The figure shows three views and two pictorial views of one solid part (mm, origin at its lowest corner). Answer the questions. A direction names the side the tool comes from. Coordinates: 2 decimals unless noted, no trailing zeros. Loops run counter-clockwise (first coordinate to the right, second up) from the corner with the lowest first, then second, coordinate; pieces in that order, holes last. Notation, with made-up numbers: M 72.25,32 L 80.25,32 A20 cw 80.25,60 Z; hole C 81,-8.5 d11. An arc over 180 degrees is marked long. One line per item, written item: value. Start each with the question number.
1. The part is cut by section A-A (y = 40.5). Write down the section's boundary in (x, z), then the cut area to 3 significant figures.
2. The part is cut by section B-B (z = 57.5). Write down the section's boundary in (x, y).
3. Consider probe 1 along X at (y, z) = (5.5, 34.5). Determine where the line is inside the solid, lowest interval first.
4. Flat-ended cylindrical pins translate along their axes: pin 1 (24 mm diameter, centred on y = 28.5, z = 66.5, fed in from -X); pin 2 (1.2 mm diameter, centred on x = 81, y = 34.5, fed in from +Z); pin 3 (14.5 mm diameter, centred on y = 39, z = 70, fed in from +X). Find the tip coordinate at first contact, or state that the pin passes through.
5. For the marked faces 1, 2 and 3, determine the directions among +Z, -Z, +X, -X, +Y, -Y from which every point of the face is accessible in a straight line to the end or side of a thin tool.
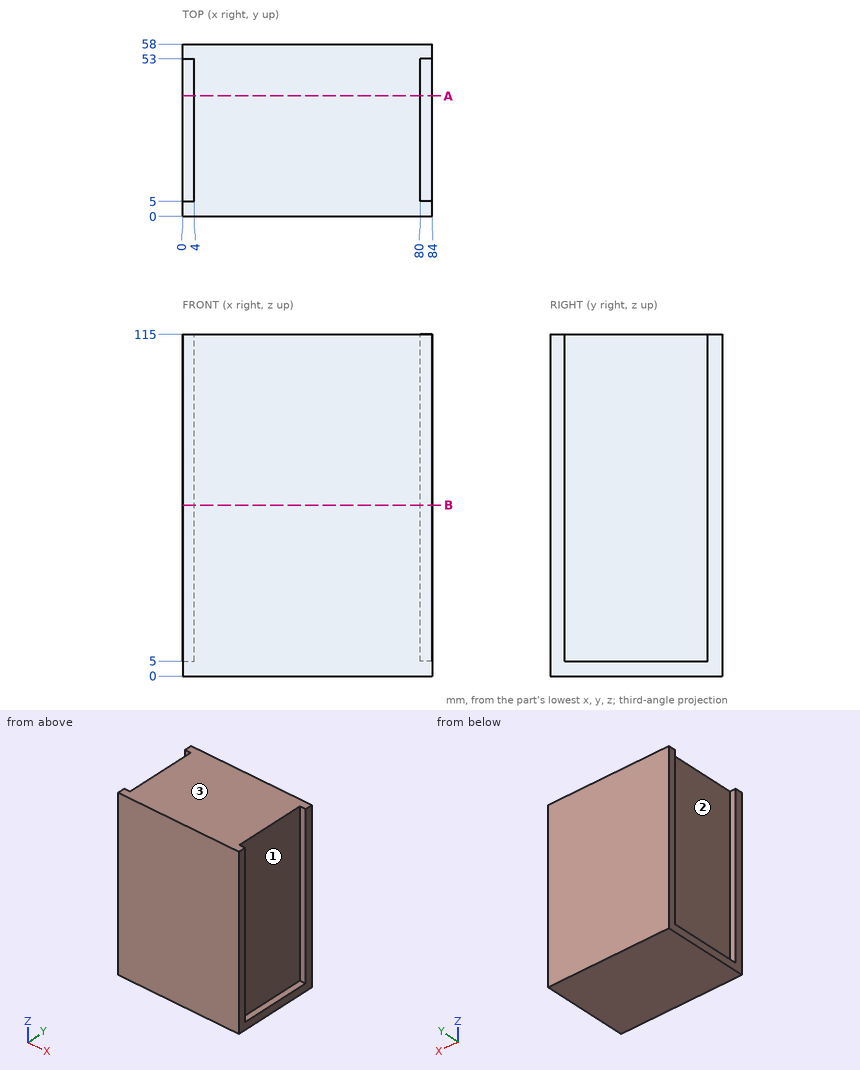
Answer block:
1. outline: M 0,0 L 84,0 L 84,5 L 80,5 L 80,115 L 4,115 L 4,5 L 0,5 Z
1. area: 8,780 mm2
2. outline: M 0,0 L 84,0 L 84,5 L 80,5 L 80,53 L 84,53 L 84,58 L 0,58 L 0,53 L 4,53 L 4,5 L 0,5 Z
3. probe 1: x = 4 to 80
4. pin 1: stops at x = 4
4. pin 2: stops at z = 5
4. pin 3: stops at x = 80
5. face 1: +Z, +X
5. face 2: +Z, -X
5. face 3: +Z, +X, -X, +Y, -Y
